Verification items for this drawing (mm, ordinates from the low corner). A direction names the side the tool comes from. Round coordinates to 2 decimals unless told otherwise and drop trailing zeros. Write each loop counter-clockwise with the first axis right and the second up, starting at its lowest first coordinate (ties: lowest second). Pieces come first, ordered by that corner, then holes.
Item 1: Access from +Z, -Z, +X, -X, +Y, -Y to the whole of each face (thin tool, end or side, straight path). Record for the marked faces 4, 5, 6, 7 and 8.
Item 2: Cross-section at A-A (y = 16). Enter the section's corners in (x, z).
Item 3: Draft check along Z on the marked faces 1, 2 and 3. Enter one of: pulls with the +Z half, pulls with the -Z half, needs draft (parallel to the pull), parting line crosses it, or undercut.
Item 4: Scan lines: probe 1 along X at (y, z) = (18.4, 6); probe 2 along Z at (x, y) = (42, 4); probe 3 along X at (y, z) = (10.5, 32). Record each from-to range of solid material in increasing order.
Item 5: Cross-section at B-B (z = 6). Enter the section's corners in (x, y).
Item 6: Cross-section at C-C (x = 22.5). Enter the section's corners in (y, z).
Item 7: Cross-section at D-D (y = 19.75). Enter the section's corners in (x, z), then the cut area to 3 significant figures.
Item 8: Depth check by flat-ended pin: P1, Ø6, axis at y = 19, z = 6.5, coming from the -X side; P2, Ø3.5, axis at x = 7.5, z = 31.5, coming from the +Y side; P3, Ø1.6, axis at x = 20, y = 20, coming from the +Z side; P4, Ø7, axis at x = 33, z = 14, coming from the -Y side. Enter the tip coordinate at first touch or a pass-through.
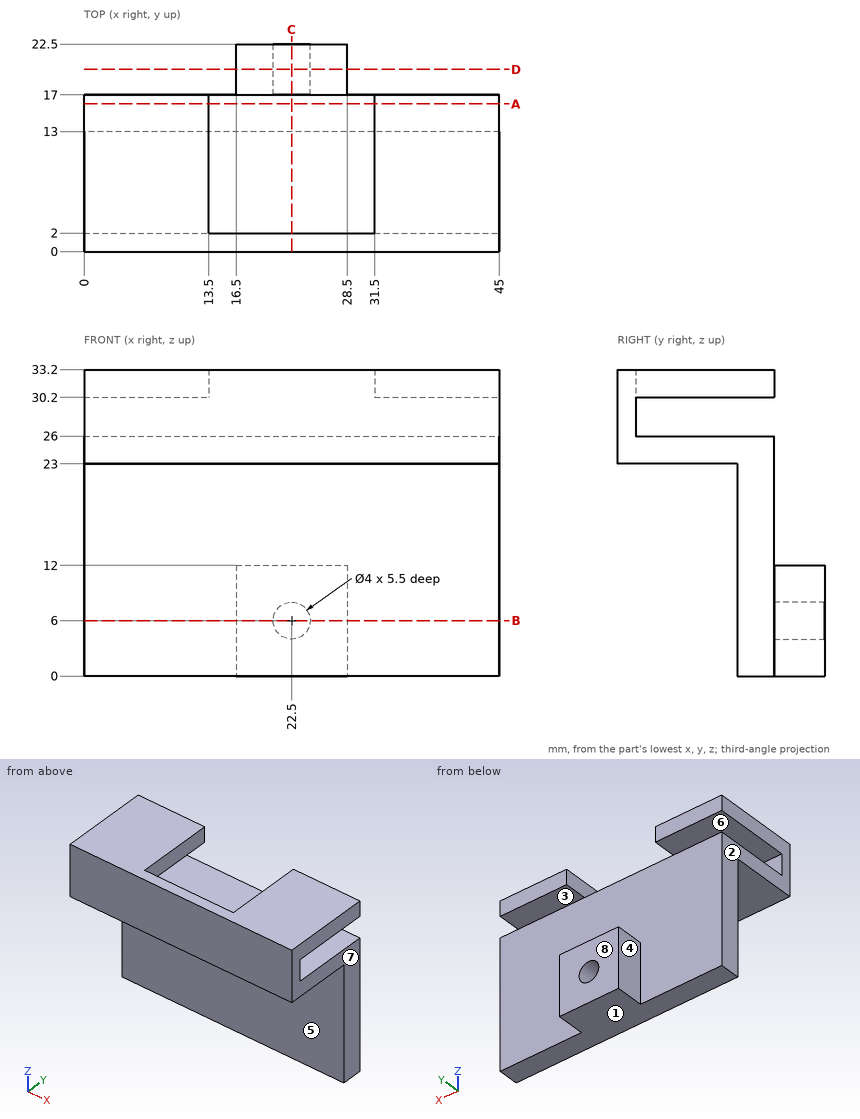
Resolved:
1. face 4: +Z, -Z, -X, +Y
1. face 5: -Z, +X, -X, -Y
1. face 6: +X, -X, +Y
1. face 7: +Z, -Z, +X, +Y, -Y
1. face 8: +Z, -Z, +X, -X, +Y
2. outline: (0, 0) - (45, 0) - (45, 26) - (0, 26) - close; (0, 30.2) - (13.5, 30.2) - (13.5, 33.2) - (0, 33.2) - close; (31.5, 30.2) - (45, 30.2) - (45, 33.2) - (31.5, 33.2) - close
3. face 1: pulls with the -Z half
3. face 2: needs draft
3. face 3: undercut
4. probe 1: x = 16.5 to 20.5, 24.5 to 28.5
4. probe 2: z = 23 to 26, 30.2 to 33.2
4. probe 3: x = 0 to 13.5, 31.5 to 45
5. outline: (0, 13) - (45, 13) - (45, 17) - (28.5, 17) - (28.5, 22.5) - (24.5, 22.5) - (24.5, 17) - (20.5, 17) - (20.5, 22.5) - (16.5, 22.5) - (16.5, 17) - (0, 17) - close
6. outline: (0, 23) - (13, 23) - (13, 0) - (22.5, 0) - (22.5, 4) - (17, 4) - (17, 8) - (22.5, 8) - (22.5, 12) - (17, 12) - (17, 26) - (2, 26) - (2, 33.2) - (0, 33.2) - close
7. outline: (16.5, 0) - (28.5, 0) - (28.5, 12) - (16.5, 12) - close; hole circle Ø4 at (22.5, 6)
7. area: 131 mm2
8. P1: stops at x = 0
8. P2: stops at y = 17
8. P3: stops at z = 12
8. P4: stops at y = 13
